Check sheet for the modelled part. Datum: model origin and axes. Units: mm. Face numbers are marked on the shaded views. A direction names the side the tool comes from. Give positions to 0.01 mm unless a question says otherwise; leave off trailing zeros. Order: outer loops, then holes, each group sorted by start corner. A loop starts at its lowest first (then second) coordinate and runs counter-clockwise, first axis right, second up.
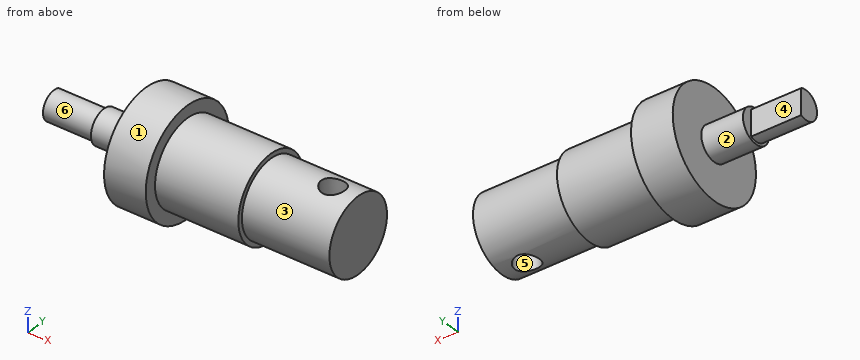
from build123d import *

# Parameters (mm, degrees)
EXTRUDE_2_DEPTH = 11
SKETCH_5_R      = 2.04
EXTRUDE_3_DEPTH = 5


with BuildPart() as part:
    # 草图1 → 旋转1 (revolve)
    with BuildSketch(Plane.XY, mode=Mode.PRIVATE) as revolve_1_sk:
        Polygon((-5, 0), (0, 0), (20.5, 0), (20.5, 4.5), (10, 4.5), (10, 5.05), (0, 5.05), (0, 6.5), (-5, 6.5), (-5, 5), align=None)
    revolve(revolve_1_sk.sketch.rotate(Axis((-5, 0, 0), (1, 0, 0)), 90), axis=Axis((-5, 0, 0), (1, 0, 0)))

    # 草图3 → 切除-旋转1 (revolve, cut)
    with BuildSketch(Plane(origin=(17.5, 0, 0), x_dir=(0, 0, -1), z_dir=(1, 0, 0)), mode=Mode.PRIVATE) as cut_revolve_1_sk:
        Polygon((-6.680542038, 0), (-6.680542038, 1.407519777), (7.599960071, 1.407519777), (7.599960071, -0.067480223), align=None)
    revolve(cut_revolve_1_sk.sketch.rotate(Axis((17.5, 0, 6.680542038), (0, -0.0047252868789963, -0.9999888357696356)), 270.416383372), axis=Axis((17.5, 0, 6.680542038), (0, -0.0047252868789963, -0.9999888357696356)), mode=Mode.SUBTRACT)

    # 草图4 → 凸台-拉伸2 (add)
    with BuildSketch(Plane.ZY.offset(5)):
        with BuildLine():
            Line((0.04652715, 0.75), (0, 0.75))
            Line((0, 0.75), (-1.547869504, 0.75))
            ThreePointArc((-1.547869504, 0.75), (0, -1.72), (1.547869504, 0.75))
            Line((1.547869504, 0.75), (0.04652715, 0.75))
        make_face()
    extrude(amount=EXTRUDE_2_DEPTH)

    # 草图5 → 凸台-拉伸3 (add)
    with BuildSketch(Plane.ZY.offset(5)):
        with Locations(Location((0, 0, 0), (0, 0, 180))):
            Circle(SKETCH_5_R)
    extrude(amount=EXTRUDE_3_DEPTH)


solid = part.part
1) Section check B-B, the plane x = 4. Record the cut outline in (y, z), then the cut area to 3 significant figures.
Recorded:
outline: circle Ø10.1 at (0, 0)
area: 80.1 mm2
2) Section check A-A, the plane y = 3. Record the cut outline in (x, z).
Recorded:
outline: (-5, -5.77) - (0, -5.77) - (0, -4.06) - (10, -4.06) - (10, -3.35) - (20.5, -3.35) - (20.5, 3.35) - (10, 3.35) - (10, 4.06) - (0, 4.06) - (0, 5.77) - (-5, 5.77) - close
3) Material ranges on L1, parallel to X at y = -3.5, z = 2.75; L2, parallel to Y at x = -12, z = 0; L3, parallel to X at y = 0, z = -6, recorded low to high.
Recorded:
L1: x = -5 to 20.5
L2: y = -1.72 to 0.75
L3: x = -5 to 0
4) Depth check by flat-ended pin: pin 1 Ø4 at (x, z) = (9.5, 4.5) entering from -Y; pin 2 Ø6 at (y, z) = (4, -2.5) entering from -X; pin 3 Ø4 at (x, y) = (-9.5, -3) entering from -Z. Enter the tip coordinate at first touch or a pass-through.
Recorded:
pin 1: stops at y = -4.39
pin 2: stops at x = -10
pin 3: stops at z = -1.78
5) Section check D-D, the plane y = 5.75. Record the cut outline in (x, z).
Recorded:
outline: (-5, -3.03) - (0, -3.03) - (0, 3.03) - (-5, 3.03) - close
6) Draft check along Y on the marked faces 4, 5 and 6. Enter one of: +Y half, -Y half, draft (parallel to the pull), parting line (faces both ways), or undercut.
Recorded:
face 4: +Y half
face 5: undercut
face 6: parting line
7) Set-up check for the marked faces 1, 2 and 3: record each of +Z, -Z, +X, -X, +Y, -Y from which the full face is reachable in a straight line by a thin tool's end or side.
Recorded:
face 1: +X, -X
face 2: -X
face 3: +X
8) Section check C-C, the plane x = 13. Record the cut outline in (y, z), then the cut area to 3 significant figures.
Recorded:
outline: circle Ø9 at (0, 0)
area: 63.6 mm2
